Can you work these out from the model? Positions are in its coordinate system, mm. Face numbers are marked on the shaded views. Round coordinates to 2 decimals unless told otherwise and drop trailing zeros. Order: outer loops, then holes, each group sorted by start corner. A loop starts at its lowest first (then second) coordinate and runs counter-clockwise, first axis right, second up.
Q1. We'd pull the mould along Y, two halves only. Please class the marked faces 1, 2 and 3: pulls with the +Y half, pulls with the -Y half, needs draft (parallel to the pull), parting line crosses it, or undercut.
Q2. If we section it at B-B (z = 4.1): Count the separate pieces of the cut face and the enclosed holes in it, plus the area to 3 significant figures.
Q3. If I drill on line 1 (Y direction, x = 35, z = 2.1); line 2 (Y direction, x = 0, z = 1.5); line 3 (X direction, y = -2.5, z = 0.45), over which ranges is the centre line in solid material (lowest first)?
Q4. If we section it at A-A (x = 0): Please give me the cut outline in (y, z), plus the area to 3 significant figures.
Q5. If we section it at C-C (y = 10): Please give me the cut outline in (x, z), plus the area to 3 significant figures.
Q6. Will these pins go through, and if not, where does the flat tip stop? P1, Ø1.9, axis at x = -25, y = 25, coming from the -Z side; P2, Ø5, axis at x = -25, y = -25, coming from the +Z side.
from build123d import *

# Parameters (mm, degrees)
SKETCH1_R           = 27.6
SKETCH1_R_2         = 2.6
BOSS_EXTRUDE1_DEPTH = 6
SKETCH4_R           = 1.6
CUT_EXTRUDE2_DEPTH  = 54.488316481
CUT_EXTRUDE3_DEPTH  = 2.5


with BuildPart() as part:
    # Sketch1 → Boss-Extrude1 (new body)
    with BuildSketch(Plane.XY):
        with BuildLine():
            Line((-35, 35), (35, 35))
            ThreePointArc((35, 35), (38.535533906, 33.535533906), (40, 30))
            Line((40, 30), (40, -30))
            ThreePointArc((40, -30), (38.535533906, -33.535533906), (35, -35))
            Line((35, -35), (-35, -35))
            ThreePointArc((-35, -35), (-38.535533906, -33.535533906), (-40, -30))
            Line((-40, -30), (-40, 30))
            ThreePointArc((-40, 30), (-38.535533906, 33.535533906), (-35, 35))
        make_face()
        Circle(SKETCH1_R, mode=Mode.SUBTRACT)
        with Locations((-35, 30)):
            Circle(SKETCH1_R_2, mode=Mode.SUBTRACT)
        with Locations((-35, -30)):
            Circle(SKETCH1_R_2, mode=Mode.SUBTRACT)
        with Locations((35, -30)):
            Circle(SKETCH1_R_2, mode=Mode.SUBTRACT)
        with Locations((35, 30)):
            Circle(SKETCH1_R_2, mode=Mode.SUBTRACT)
    extrude(amount=BOSS_EXTRUDE1_DEPTH)

    # Sketch4 → Cut-Extrude2 (cut, through all)
    with BuildSketch(Plane(origin=(0, 0, 0), x_dir=(-1, 0, 0), z_dir=(0, 0, -1))):
        with Locations((-25, 25)):
            Circle(SKETCH4_R)
        with Locations((25, 25)):
            Circle(SKETCH4_R)
        with Locations((-25, -25)):
            Circle(SKETCH4_R)
        with Locations((25, -25)):
            Circle(SKETCH4_R)
    extrude(amount=-CUT_EXTRUDE2_DEPTH, mode=Mode.SUBTRACT)

    # Sketch5 → Cut-Extrude3 (cut)
    with BuildSketch(Plane(origin=(0, 0, 0), x_dir=(-1, 0, 0), z_dir=(0, 0, -1))):
        Polygon((-28.290896534, 25), (-26.645448267, 22.15), (-23.354551733, 22.15), (-21.709103466, 25), (-23.354551733, 27.85), (-26.645448267, 27.85), align=None)
        Polygon((21.709103466, 25), (23.354551733, 22.15), (26.645448267, 22.15), (28.290896534, 25), (26.645448267, 27.85), (23.354551733, 27.85), align=None)
        Polygon((-28.29088256, -24.990409574), (-26.653746833, -27.845192685), (-23.362864273, -27.854783111), (-21.70911744, -25.009590426), (-23.346253167, -22.154807315), (-26.637135727, -22.145216889), align=None)
        Polygon((28.290801988, -24.975054549), (26.6237976, -22.137609154), (23.332995612, -22.162554605), (21.709198012, -25.024945451), (23.3762024, -27.862390846), (26.667004388, -27.837445395), align=None)
    extrude(amount=-CUT_EXTRUDE3_DEPTH, mode=Mode.SUBTRACT)


solid = part.part
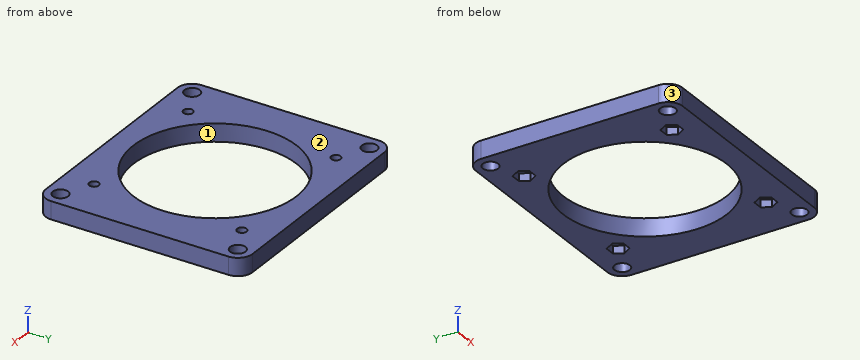
Solution:
1. face 1: undercut
1. face 2: needs draft
1. face 3: pulls with the -Y half
2. separate pieces: 1
2. enclosed holes: 9
2. area: 3,070 mm2
3. line 1: y = -35 to -32.6, -27.4 to 27.4, 32.6 to 35
3. line 2: y = -35 to -27.6, 27.6 to 35
3. line 3: x = -40 to -27.49, 27.49 to 40
4. outline: (-35, 0) - (-27.6, 0) - (-27.6, 6) - (-35, 6) - close; (27.6, 0) - (35, 0) - (35, 6) - (27.6, 6) - close
4. area: 88.8 mm2
5. outline: (-40, 0) - (-25.72, 0) - (-25.72, 6) - (-40, 6) - close; (25.72, 0) - (40, 0) - (40, 6) - (25.72, 6) - close
5. area: 171 mm2
6. P1: passes through
6. P2: stops at z = 6
